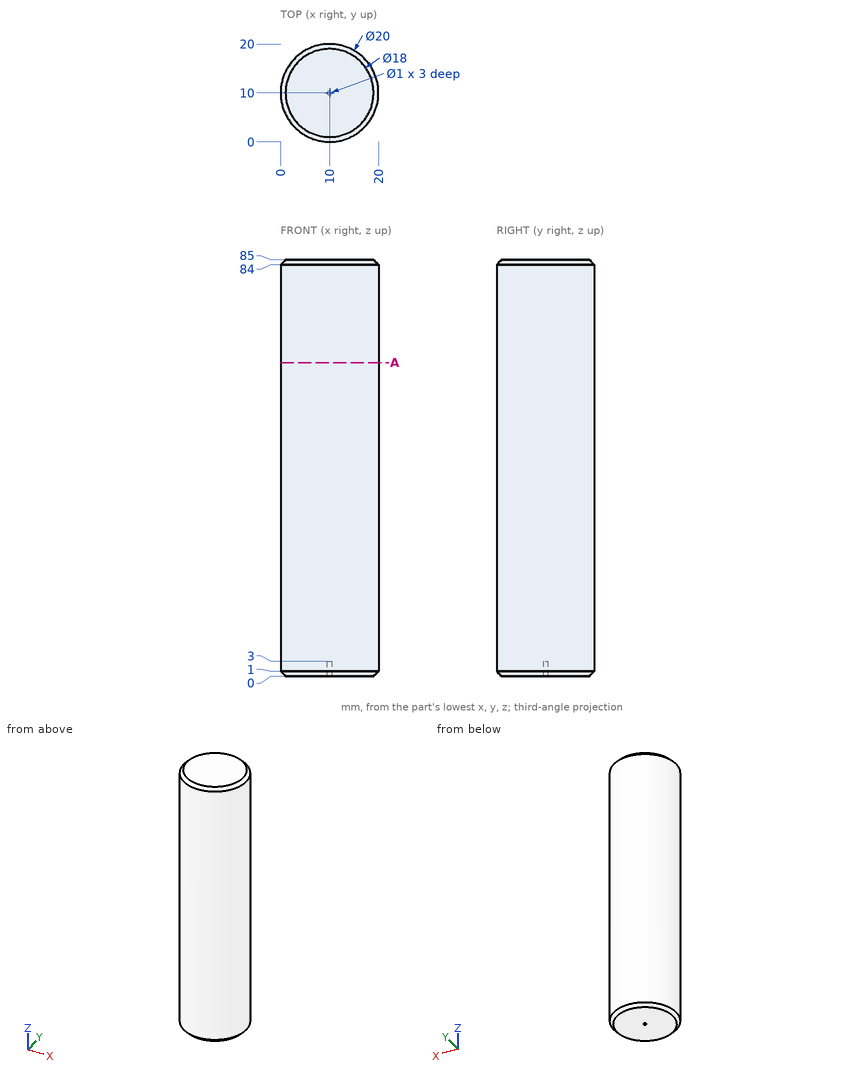
Drawing for the job (mm, zero at the part's lowest x, y, z). Coordinates: 2 decimals unless noted, no trailing zeros. Order: outer loops, then holes, each group sorted by start corner. A loop starts at its lowest first (then second) coordinate and runs counter-clockwise, first axis right, second up. Notation, with made-up numbers: (-36, 21) -> (7, 21) arc R24 cw to (7, 47) -> close; hole circle Ø7 at (18, 83.5). An arc over 180 degrees is marked (long way). Answer in a Markdown table with one row per item.
1) Drill centre lines: line 1 (Y direction, x = 10, z = 1.25); line 2 (Y direction, x = 10, z = 0.9); line 3 (X direction, y = 3.75, z = 11). Where is each one in solid material? Low to high.
Check values:
| item | result |
|---|---|
| line 1 | 0 to 9.5, 10.5 to 20 |
| line 2 | 0.1 to 9.5, 10.5 to 19.9 |
| line 3 | 2.19 to 17.81 |
2) Band-saw the part on A-A (z = 64). List the corners of the cut face in (x, y).
Check values:
| item | result |
|---|---|
| outline | circle Ø20 at (10, 10) |
3) Flat gauge pins, fed straight in: P1, Ø6, axis at x = 14.5, z = 13.5, coming from the +Y side; P2, Ø0.5, axis at x = 10, y = 10, coming from the -Z side; P3, Ø5, axis at y = 16, z = 54, coming from the -X side. Where does each tip first touch, or does it go through?
Check values:
| item | result |
|---|---|
| P1 | y = 19.89 |
| P2 | z = 3 |
| P3 | x = 0.63 |
